The listing builds one solid part. Answer for the finished solid, in the listing's coordinates (mm). Coordinates: 2 decimals unless noted, no trailing zeros. Write each loop counter-clockwise with the first axis right and the second up, starting at its lowest first coordinate (ties: lowest second). Pieces come first, ordered by that corner, then holes.
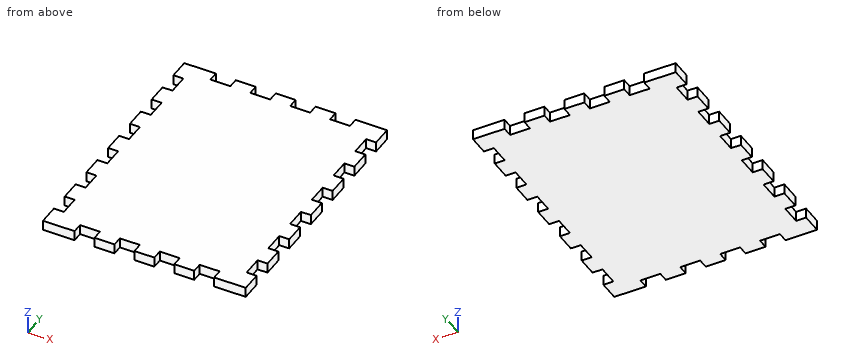
from build123d import *

# Parameters (mm, degrees)
EXTRUDE_1_DEPTH = 3


with BuildPart() as part:
    # 草图2 → 凸台-拉伸1 (new body)
    with BuildSketch(Plane.XY):
        Polygon((0, 81), (0, 75), (3, 75), (3, 69), (0, 69), (0, 63), (3, 63), (3, 57), (0, 57), (0, 51), (3, 51), (3, 45), (0, 45), (0, 39), (3, 39), (3, 33), (0, 33), (0, 27), (3, 27), (3, 21), (0, 21), (0, 15), (3, 15), (3, 9), (0, 9), (0, 3), (9.5, 3), (9.5, 6), (15.5, 6), (15.5, 3), (21.5, 3), (21.5, 6), (27.5, 6), (27.5, 3), (33.5, 3), (33.5, 6), (39.5, 6), (39.5, 3), (45.5, 3), (45.5, 6), (51.5, 6), (51.5, 3), (57.5, 3), (61, 3), (61, 9), (58, 9), (58, 15), (61, 15), (61, 21), (58, 21), (58, 27), (61, 27), (61, 33), (58, 33), (58, 39), (61, 39), (61, 45), (58, 45), (58, 51), (61, 51), (61, 57), (58, 57), (58, 63), (61, 63), (61, 69), (58, 69), (58, 75), (61, 75), (61, 81), (51.5, 81), (51.5, 78), (45.5, 78), (45.5, 81), (39.5, 81), (39.5, 78), (33.5, 78), (33.5, 81), (27.5, 81), (27.5, 78), (21.5, 78), (21.5, 81), (15.5, 81), (15.5, 78), (9.5, 78), (9.5, 81), (3.5, 81), align=None)
    extrude(amount=EXTRUDE_1_DEPTH)


solid = part.part
1. Flat-ended cylindrical pins translate along their axes: P1, Ø0.9, axis at x = 48.5, z = 1.5, coming from the +Y side; P2, Ø1.5, axis at x = 13.5, z = 2, coming from the -Y side; P3, Ø0.9, axis at y = 13, z = 2, coming from the -X side. Find the tip coordinate at first contact, or state that the pin passes through.
Results found:
P1: stops at y = 78
P2: stops at y = 6
P3: stops at x = 3
2. Find the intervals of material crossed by L1, parallel to X at y = 73, z = 2.3; L2, parallel to Y at x = 35, z = 2.15, in increasing order.
Results found:
L1: x = 3 to 58
L2: y = 6 to 78
3. Section A-A on x = 35.5 is taken. Give the vertices of the cut face in (y, z), then the cut area to 3 significant figures.
Results found:
outline: (6, 0) - (78, 0) - (78, 3) - (6, 3) - close
area: 216 mm2
